from build123d import *

# Parameters (mm, degrees)
SKETCH1_R           = 1.6
SKETCH1_R_2         = 2.5
BOSS_EXTRUDE1_DEPTH = 5
FILLET1_R           = 1.5
CUT_EXTRUDE1_START  = -10
CUT_EXTRUDE1_DEPTH  = 10
FILLET2_R           = 3
BOSS_EXTRUDE2_DEPTH = 5
CHAMFER1_SIZE2      = 8.660254038
CHAMFER1_SIZE       = 5
CHAMFER2_SIZE2      = 5
CHAMFER2_SIZE       = 8.660254038


# Some blends are built 0.0001 mm under size
with BuildPart() as part:
    # Sketch1 → Boss-Extrude1 (new body)
    with BuildSketch(Plane(origin=(0, 0, 0), x_dir=(1, 0, 0), z_dir=(0, 1, 0))):
        with BuildLine():
            ThreePointArc((-85.12409805, 73.840708631), (-84.725396744, 73.411688245), (-84.296376359, 73.012986939))
            ThreePointArc((-84.296376359, 73.012986939), (-83.127079594, 65.649461526), (-75.690864757, 65.109581606))
            Line((-75.690864757, 65.109581606), (-28.156854249, 17.575571099))
            ThreePointArc((-28.156854249, 17.575571099), (-17.196699141, 17.196699141), (-17.575571099, 28.156854249))
            Line((-17.575571099, 28.156854249), (-65.109581606, 75.690864757))
            ThreePointArc((-65.109581606, 75.690864757), (-65.649461526, 83.127079594), (-73.012986939, 84.296376359))
            ThreePointArc((-73.012986939, 84.296376359), (-73.411688245, 84.725396744), (-73.840708631, 85.12409805))
            ThreePointArc((-73.840708631, 85.12409805), (-79.068542495, 94.068542495), (-84.296376359, 85.12409805))
            ThreePointArc((-84.296376359, 85.12409805), (-84.725396744, 84.725396744), (-85.12409805, 84.296376359))
            ThreePointArc((-85.12409805, 84.296376359), (-94.068542495, 79.068542495), (-85.12409805, 73.840708631))
        make_face()
        with BuildLine():
            Line((-80.668542495, 86.068542495), (-80.668542495, 88.068542495))
            ThreePointArc((-80.668542495, 88.068542495), (-79.068542495, 89.668542495), (-77.468542495, 88.068542495))
            Line((-77.468542495, 88.068542495), (-77.468542495, 86.068542495))
            ThreePointArc((-77.468542495, 86.068542495), (-79.068542495, 84.468542495), (-80.668542495, 86.068542495))
        make_face(mode=Mode.SUBTRACT)
        with Locations(Location((-22.5, 22.5, 0), (0, 0, 270))):
            Circle(SKETCH1_R, mode=Mode.SUBTRACT)
        with Locations(Location((-32.5, 32.5, 0), (0, 0, 270))):
            Circle(SKETCH1_R, mode=Mode.SUBTRACT)
        with BuildLine():
            Line((-80.668542495, 70.068542495), (-80.668542495, 72.068542495))
            ThreePointArc((-80.668542495, 72.068542495), (-79.068542495, 73.668542495), (-77.468542495, 72.068542495))
            Line((-77.468542495, 72.068542495), (-77.468542495, 70.068542495))
            ThreePointArc((-77.468542495, 70.068542495), (-79.068542495, 68.468542495), (-80.668542495, 70.068542495))
        make_face(mode=Mode.SUBTRACT)
        with BuildLine():
            Line((-86.068542495, 77.468542495), (-88.068542495, 77.468542495))
            ThreePointArc((-88.068542495, 77.468542495), (-89.668542495, 79.068542495), (-88.068542495, 80.668542495))
            Line((-88.068542495, 80.668542495), (-86.068542495, 80.668542495))
            ThreePointArc((-86.068542495, 80.668542495), (-84.468542495, 79.068542495), (-86.068542495, 77.468542495))
        make_face(mode=Mode.SUBTRACT)
        with Locations(Location((-79.068542495, 79.068542495, 0), (0, 0, 270))):
            Circle(SKETCH1_R_2, mode=Mode.SUBTRACT)
        with BuildLine():
            ThreePointArc((-70.068542495, 80.668542495), (-68.468542495, 79.068542495), (-70.068542495, 77.468542495))
            Line((-70.068542495, 77.468542495), (-72.068542495, 77.468542495))
            ThreePointArc((-72.068542495, 77.468542495), (-73.668542495, 79.068542495), (-72.068542495, 80.668542495))
            Line((-72.068542495, 80.668542495), (-70.068542495, 80.668542495))
        make_face(mode=Mode.SUBTRACT)
    extrude(amount=BOSS_EXTRUDE1_DEPTH)

    # Fillet1
    # the kernel refuses this fillet: 1.5 mm, written as the material it adds along each edge
    with BuildSketch(Plane(origin=(-75.690864757, 0, -65.109581606), x_dir=(-0.8710919006324759, 0, 0.4911200470887958), z_dir=(0, 1, 0))) as fillet1_piece_1:
        with BuildLine():
            CenterArc((1.140350885, 1.494638979), FILLET1_R, 195.585774364, 69.56865207)
            Line((-0.304493073, 1.091617967), (0, 0))
            ThreePointArc((0, 0), (0.506822616, 0.021444084), (1.013645231, 0))
        make_face()
    extrude(amount=5)
    with BuildSketch(Plane(origin=(-65.109581606, 0, -75.690864757), x_dir=(0.70710678118656, 0, 0.7071067811865349), z_dir=(0, 1, 0))) as fillet1_piece_2:
        with BuildLine():
            CenterArc((1.133289821, 1.5), FILLET1_R, 200.43134793, 69.56865207)
            ThreePointArc((-0.272346884, 0.976372792), (-0.115517872, 0.493948007), (0, 0))
            Line((0, 0), (1.133289821, 0))
        make_face()
    extrude(amount=5)
    with BuildSketch(Plane(origin=(-84.296376359, 0, -85.12409805), x_dir=(-0.7160400781456726, 0, 0.6980591711947771), z_dir=(0, 1, 0))) as fillet1_piece_3:
        with BuildLine():
            CenterArc((1.058307083, -1.497254596), FILLET1_R, 93.467060005, 62.635531643)
            ThreePointArc((-0.313101337, -0.889604248), (-0.139044818, -0.450963409), (0, 0))
            ThreePointArc((0, 0), (0.483797523, -0.014642152), (0.967595047, 0))
        make_face()
    extrude(amount=5)
    with BuildSketch(Plane(origin=(-73.840708631, 0, -85.12409805), x_dir=(0.7160400781456655, 0, 0.6980591711947844), z_dir=(0, 1, 0)), Plane(origin=(-85.12409805, 0, -84.296376359), x_dir=(0.698059171194804, 0, -0.7160400781456464), z_dir=(0, 1, 0)), Plane(origin=(-84.296376359, 0, -73.012986939), x_dir=(-0.716040078145762, 0, -0.6980591711946854), z_dir=(0, 1, 0))) as fillet1_piece_4:
        with BuildLine():
            CenterArc((1.058307083, 1.497254596), FILLET1_R, 203.897408353, 62.635531643)
            ThreePointArc((-0.313101337, 0.889604248), (-0.139044818, 0.450963409), (0, 0))
            ThreePointArc((0, 0), (0.483797523, 0.014642152), (0.967595047, 0))
        make_face()
    extrude(amount=5)
    with BuildSketch(Plane(origin=(-73.012986939, 0, -84.296376359), x_dir=(0.9071785576189849, 0, -0.42074584323120545), z_dir=(0, 1, 0)), Plane(origin=(-85.12409805, 0, -73.840708631), x_dir=(-0.9071785576191526, 0, 0.4207458432308441), z_dir=(0, 1, 0))) as fillet1_piece_5:
        with BuildLine():
            CenterArc((1.060981867, 1.495360386), FILLET1_R, 202.856873055, 62.635531643)
            ThreePointArc((-0.321235194, 0.912714701), (-0.146805923, 0.461218449), (0, 0))
            ThreePointArc((0, 0), (0.471547497, 0.018558455), (0.943094993, 0))
        make_face()
    extrude(amount=5)

    # Sketch4 → Cut-Extrude1 (cut)
    with BuildSketch(Plane(origin=(0, 5, 0), x_dir=(1, 0, 0), z_dir=(0, 1, 0)).offset(CUT_EXTRUDE1_START)):
        with BuildLine():
            Line((-15.011619019, 22.917313169), (-18.964466094, 18.964466094))
            Line((-18.964466094, 18.964466094), (-17.196699141, 17.196699141))
            ThreePointArc((-17.196699141, 17.196699141), (-15.493707308, 19.823834327), (-15.011619019, 22.917313169))
        make_face()
        with BuildLine():
            Line((-17.196699141, 17.196699141), (-18.964466094, 18.964466094))
            Line((-18.964466094, 18.964466094), (-22.917313169, 15.011619019))
            ThreePointArc((-22.917313169, 15.011619019), (-19.823834327, 15.493707308), (-17.196699141, 17.196699141))
        make_face()
    extrude(amount=CUT_EXTRUDE1_DEPTH, mode=Mode.SUBTRACT)

    # Fillet2
    fillet2_edges = [part.edges().sort_by_distance(p)[0] for p in [
        (-22.917313169, 2.5, -15.011619019),
        (-15.011619019, 2.5, -22.917313169),
    ]]
    fillet(fillet2_edges, radius=FILLET2_R)

    # Sketch5 → Boss-Extrude2 (add)
    with BuildSketch(Plane.XZ):
        Polygon((-70.70206426, -64.910255721), (-67.806159991, -67.806159991), (-39.521888743, -39.521888743), (-42.417793012, -36.625984474), align=None)
        Polygon((-39.521888743, -39.521888743), (-67.806159991, -67.806159991), (-65.04521001, -70.567109971), (-36.760938763, -42.282838723), align=None)
    extrude(amount=BOSS_EXTRUDE2_DEPTH)

    # Chamfer1
    chamfer1_edges = [part.edges().sort_by_distance(p)[0] for p in [
        (-67.873637135, -5, -67.738682846),
    ]]
    chamfer1_side = [part.faces().sort_by_distance(p)[0] for p in [
        (-67.873637135, -4.9, -67.738682846),
    ]]
    chamfer(chamfer1_edges, length=CHAMFER1_SIZE - 0.0001, length2=CHAMFER1_SIZE2 - 0.0001, reference=chamfer1_side[0])  # a hair under: the kernel refuses the full size

    # Chamfer2
    chamfer2_edges = [part.edges().sort_by_distance(p)[0] for p in [
        (-39.589365887, -5, -39.454411599),
    ]]
    chamfer2_side = [part.faces().sort_by_distance(p)[0] for p in [
        (-39.660076566, -5, -39.525122277),
    ]]
    chamfer(chamfer2_edges, length=CHAMFER2_SIZE - 0.0001, length2=CHAMFER2_SIZE2 - 0.0001, reference=chamfer2_side[0])  # a hair under: the kernel refuses the full size


solid = part.part
Build history of the part. All positions in model axes, mm. A direction names the side the tool comes from. Coordinates: 2 decimals unless noted, no trailing zeros. Write each loop counter-clockwise with the first axis right and the second up, starting at its lowest first coordinate (ties: lowest second). Pieces come first, ordered by that corner, then holes. Notation, with made-up numbers: (35.25, 7.25) -> (51.25, 7.25) arc R27 cw to (51.25, 26.25) -> close; hole circle Ø5 at (76, -13.5). An arc over 180 degrees is marked (long way). Use CSV: the item, a comma, the result in double quotes. Start each with the question number.
Q1. Flat gauge pins, fed straight in: pin 1 Ø0.6 at (x, y) = (-87.5, 1.5) entering from -Z; pin 2 Ø2 at (x, y) = (-26, -0.5) entering from +Z; pin 3 Ø1 at (x, y) = (-70.5, 2) entering from +Z; pin 4 Ø3 at (x, z) = (-22.5, -22.5) entering from +Y. Where does each tip first touch, or does it go through?
Q2. Cut at B-B, the plane z = -32.5. List the corners of the cut face in (x, y).
Q3. Cut at D-D, the plane y = 4. State how many separate pieces and enclosed holes the cut face has, then the cut area to 3 significant figures.
Q4. Drill centre lines: probe 1 along Z at (x, y) = (-80, 0.5); probe 2 along Y at (x, z) = (-82, -74); probe 3 along Z at (x, y) = (-69.5, 2). Where is each one in solid material? Low to high.
Q5. Cut at C-C, the plane y = -4. List the corners of the cut face in (x, z).
Q6. 3-axis set-ups, long thin cutter, end or side, ignore diameter. For faces 1 (the cylindrical face through (-73.67, 2.46, -79.03)), 2 (the flat face through (-56.36, -2.47, -50.57)), 3 (the flat face through (-56, 0, -49)): which of +Z, -Z, +X, -X, +Y, -Y reach the whole face in a straight line?
Q7. Pull direction Z, two halves, no side cores. Call faces 4 (the cylindrical face through (-15.32, 2.54, -23.23)), 5 (the cylindrical face through (-26.69, 2.46, -16.28)), 6 (the cylindrical face through (-84.47, 2.46, -79.1)): released by +Z, released by -Z, zero draft, split by the parting line, or undercut.
Q8. Cut at A-A, the plane x = -32.5. List the corners of the cut face in (y, z), then the cut area to 3 significant figures.
Checked values:
1,pin 1,"stops at z = -85.06"
1,pin 2,"stops at z = -15.48"
1,pin 3,"stops at z = -59.42"
1,pin 4,"passes through"
2,outline,"(-43.08, 0) -> (-34.1, 0) -> (-34.1, 5) -> (-43.08, 5) -> close; (-30.9, 0) -> (-21.92, 0) -> (-21.92, 5) -> (-30.9, 5) -> close"
3,separate pieces,"1"
3,enclosed holes,"7"
3,area,"1,510 mm²"
4,probe 1,"z = -94 to -89.37, -84.77 to -81.39, -76.75 to -73.37, -68.77 to -64.14"
4,probe 2,"y = 0 to 5"
4,probe 3,"z = -85.04 to -80.56, -77.57 to -58.92"
5,outline,"(-65.8, -60.01) -> (-60.15, -65.67) -> (-41.66, -47.18) -> (-47.32, -41.52) -> close"
6,face 1,"+Y, -Y"
6,face 2,"+Z, -X, -Y"
6,face 3,"-Y"
7,face 4,"split by the parting line"
7,face 5,"released by +Z"
7,face 6,"undercut"
8,outline,"(0, -43.08) -> (5, -43.08) -> (5, -34.1) -> (0, -34.1) -> close; (0, -30.9) -> (5, -30.9) -> (5, -21.92) -> (0, -21.92) -> close"
8,area,"89.8 mm²"
